Can you work these out from the model? Positions are in its coordinate system, mm. Face numbers are marked on the shaded views. A direction names the side the tool comes from. Give positions to 0.01 mm unless a question says otherwise; leave off trailing zeros. Loops run counter-clockwise (first coordinate to the right, second up) from the corner with the lowest first, then second, coordinate; pieces in that order, holes last. Notation, with made-up numbers: M 33,-6.5 L 58,-6.5 A24 ccw 58,7.5 Z; hole C 19.5,46 d8. An arc over 180 degrees is marked long. Put each result on its own line as item: value. Start each with the question number.
1) For P1, Ø8, axis at x = 21.5, y = 3.5, coming from the +Z side; P2, Ø3, axis at x = -3.5, y = 12, coming from the +Z side; P3, Ø5, axis at x = -26, z = -51, coming from the +Y side; P4, Ø2.5, axis at x = -28, z = -27.5, coming from the +Y side, each with a flat end and sliding along its axis, tell me the tip position at first contact or that it passes through.
2) If we mould it in two halves opening along X, with no side actions, what happens to the marked faces 4, 5 and 6? For each: +X half, -X half, draft (parallel to the pull), parting line (faces both ways), or undercut.
3) Please list where these lines run through material, in increasing order: line 1 along Z through (x, y) = (0, 2.75); line 2 along Z through (x, y) = (-27.5, 6.85); line 3 along Z through (x, y) = (4, 7.25). Write a range as from..to.
4) Imagine slicing it at A-A (y = 11.5). Write out the boundary of the cut face in (x, z).
5) For the marked faces 1, 2 and 3, which set-ups out of +Z, -Z, +X, -X, +Y, -Y let a thin tool reach every point of the face, with its end or its side?
6) Imagine slicing it at C-C (y = 5.25). State how many separate pieces and enclosed holes the cut face has, then the cut area to 3 significant figures.
7) Imagine slicing it at B-B (x = 18.5). Write out the boundary of the cut face in (y, z), then the cut area to 3 significant figures.
from build123d import *

# Parameters (mm, degrees)
BOSS_EXTRUDE1_DEPTH       = 7
FILLET1_R                 = 2
FILLET2_R                 = 10
SKETCH2_R                 = 10
BOSS_EXTRUDE2_DEPTH       = 8
FILLET3_R                 = 2
M10_CLEARANCE_HOLE1_D     = 10
M10_CLEARANCE_HOLE1_DEPTH = 10
M10_CLEARANCE_HOLE1_TIP   = 3.004303095
M5X0_8_TAPPED_HOLE1_D     = 4.2
M5X0_8_TAPPED_HOLE1_DEPTH = 12.4
M5X0_8_TAPPED_HOLE1_TIP   = 1.2618073
SKETCH6_R                 = 4.65
CUT_EXTRUDE1_DEPTH        = 0.55
SKETCH8_R                 = 4.65
CUT_EXTRUDE2_DEPTH        = 0.55
SKETCH9_R                 = 2.5
SKETCH10_R                = 4.65
CUT_EXTRUDE3_DEPTH        = 0.55
SKETCH11_R                = 2.5
SKETCH12_R                = 4.65
CUT_EXTRUDE4_DEPTH        = 0.55
SKETCH13_R                = 2.5


with BuildPart() as part:
    # Sketch1 → Boss-Extrude1 (new body)
    with BuildSketch(Plane(origin=(0, 0, 0), x_dir=(1, 0, 0), z_dir=(0, 1, 0))):
        with BuildLine():
            Line((-29, 35.312691864), (-29, 61.312691864))
            ThreePointArc((-29, 61.312691864), (-35.104593263, 71.654789625), (-24.072111437, 76.399195782))
            ThreePointArc((-24.072111437, 76.399195782), (0, 91.170808686), (24.072111437, 76.399195782))
            ThreePointArc((24.072111437, 76.399195782), (35.104593263, 71.654789625), (29, 61.312691864))
            Line((29, 61.312691864), (29, 35.312691864))
            ThreePointArc((29, 35.312691864), (35.126764687, 25.039526301), (24.203518415, 20.16532205))
            ThreePointArc((24.203518415, 20.16532205), (0, 5.30985101), (-24.203518415, 20.16532205))
            ThreePointArc((-24.203518415, 20.16532205), (-35.126764687, 25.039526301), (-29, 35.312691864))
        make_face()
    extrude(amount=BOSS_EXTRUDE1_DEPTH)

    # Fillet1
    fillet1_edges = [part.edges().sort_by_distance(p)[0] for p in [
        (29, 3.5, -61.312691864),
        (29, 3.5, -35.312691864),
        (-29, 3.5, -35.312691864),
        (-29, 3.5, -61.312691864),
    ]]
    fillet(fillet1_edges, radius=FILLET1_R)

    # Fillet2
    fillet2_edges = [part.edges().sort_by_distance(p)[0] for p in [
        (24.072111437, 3.5, -76.399195782),
        (24.203518415, 3.5, -20.16532205),
        (-24.203518415, 3.5, -20.16532205),
        (-24.072111437, 3.5, -76.399195782),
    ]]
    fillet(fillet2_edges, radius=FILLET2_R)

    # Sketch2 → Boss-Extrude2 (add)
    with BuildSketch(Plane(origin=(0, 7, 0), x_dir=(1, 0, 0), z_dir=(0, 1, 0))):
        with Locations(Location((0, 64.170808686, 0), (0, 0, 270))):
            Circle(SKETCH2_R)
        with Locations(Location((0, 32.454575041, 0), (0, 0, 270))):
            Circle(SKETCH2_R)
    extrude(amount=BOSS_EXTRUDE2_DEPTH)

    # Fillet3
    fillet3_edges = [part.edges().sort_by_distance(p)[0] for p in [
        (0, 7, -74.170808686),
        (0, 15, -74.170808686),
        (0, 7, -42.454575041),
        (0, 15, -42.454575041),
    ]]
    fillet(fillet3_edges, radius=FILLET3_R)

    # M10 Clearance Hole1
    with Locations(Plane(origin=(0, 0, -32.454575041), x_dir=(0, 0, -1), z_dir=(0, -1, 0))):
        with Locations((0, 0), (31.716233645, 0)):
            Hole(M10_CLEARANCE_HOLE1_D / 2, depth=M10_CLEARANCE_HOLE1_DEPTH)
            with Locations((0, 0, -(M10_CLEARANCE_HOLE1_DEPTH + M10_CLEARANCE_HOLE1_TIP / 2))):  # 118° drill point
                Cone(0, M10_CLEARANCE_HOLE1_D / 2, M10_CLEARANCE_HOLE1_TIP, mode=Mode.SUBTRACT)

    # M5x0.8 Tapped Hole1
    with Locations(Plane(origin=(-27.5, 7, -69.170808686), x_dir=(0, 0, 1), z_dir=(0, 1, 0))):
        with Locations((0, 0), (0, 55), (41.716233645, 55), (41.716233645, 0)):
            Hole(M5X0_8_TAPPED_HOLE1_D / 2, depth=M5X0_8_TAPPED_HOLE1_DEPTH)
            with Locations((0, 0, -(M5X0_8_TAPPED_HOLE1_DEPTH + M5X0_8_TAPPED_HOLE1_TIP / 2))):  # 118° drill point
                Cone(0, M5X0_8_TAPPED_HOLE1_D / 2, M5X0_8_TAPPED_HOLE1_TIP, mode=Mode.SUBTRACT)

    # Sketch6 → Cut-Extrude1 (cut)
    with BuildSketch(Plane(origin=(0, 7, 0), x_dir=(1, 0, 0), z_dir=(0, 1, 0))):
        with Locations(Location((27.5, 69.170808686, 0), (0, 0, 270))):
            Circle(SKETCH6_R)
    extrude(amount=-CUT_EXTRUDE1_DEPTH, mode=Mode.SUBTRACT)

    # Cut-Loft1: read off the stored shape, not the designer's step
    # Cut-Loft1: loft between two sections, ruled curve by curve
    cut_loft1_from = [
        Edge.make_bspline([(25.414803916, 4.3, -70.549923363), (22.656574563, 4.3, -66.379531195), (26.826966731, 4.3, -63.621301842), (29.585196084, 4.3, -67.79169401), (32.343425437, 4.3, -71.962086178), (28.173033269, 4.3, -74.720315531), (25.414803916, 4.3, -70.549923363)], [0, 0, 0, 0, 0.5, 0.5, 0.5, 1, 1, 1, 1], 3, [1, 0.333333333, 0.333333333, 1, 0.333333333, 0.333333333, 1]),
    ]
    cut_loft1_to = [
        Edge.make_bspline([(23.222066223, 6.45, -70.993384502), (19.576914593, 6.45, -62.437516949), (28.132782146, 6.45, -58.792365318), (31.777933777, 6.45, -67.348232871), (35.423085407, 6.45, -75.904100424), (26.867217854, 6.45, -79.549252055), (23.222066223, 6.45, -70.993384502)], [0, 0, 0, 0, 0.5, 0.5, 0.5, 1, 1, 1, 1], 3, [1, 0.333333333, 0.333333333, 1, 0.333333333, 0.333333333, 1]),
    ]
    cut_loft1 = Solid(Shell([*[Face.make_surface_from_curves(cut_loft1_from[k], cut_loft1_to[k]) for k in range(1)], Face(Wire(cut_loft1_from)), Face(Wire(cut_loft1_to))]))
    add(cut_loft1, mode=Mode.SUBTRACT)

    # Sketch8 → Cut-Extrude2 (cut)
    with BuildSketch(Plane(origin=(0, 7, 0), x_dir=(1, 0, 0), z_dir=(0, 1, 0))):
        with Locations(Location((-27.5, 69.170808686, 0), (0, 0, 270))):
            Circle(SKETCH8_R)
    extrude(amount=-CUT_EXTRUDE2_DEPTH, mode=Mode.SUBTRACT)

    # Sketch9 → section 0 of cut_loft2
    with BuildSketch(Plane(origin=(0, 4.3, 0), x_dir=(1, 0, 0), z_dir=(0, 1, 0)), mode=Mode.PRIVATE) as cut_loft2_s0:
        with Locations((-27.5, 69.170808686)):
            Circle(SKETCH9_R)
    # loft up to a face of the part (cut_loft2)
    loft([cut_loft2_s0.sketch, Face(Wire([part.edges().sort_by_distance((-24.110295882, 6.45, -72.353952729))[0]]))], mode=Mode.SUBTRACT)

    # Sketch10 → Cut-Extrude3 (cut)
    with BuildSketch(Plane(origin=(0, 7, 0), x_dir=(1, 0, 0), z_dir=(0, 1, 0))):
        with Locations(Location((-27.5, 27.454575041, 0), (0, 0, 270))):
            Circle(SKETCH10_R)
    extrude(amount=-CUT_EXTRUDE3_DEPTH, mode=Mode.SUBTRACT)

    # Sketch11 → section 0 of cut_loft3
    with BuildSketch(Plane(origin=(0, 4.3, 0), x_dir=(1, 0, 0), z_dir=(0, 1, 0)), mode=Mode.PRIVATE) as cut_loft3_s0:
        with Locations((-27.5, 27.454575041)):
            Circle(SKETCH11_R)
    # loft up to a face of the part (cut_loft3)
    loft([cut_loft3_s0.sketch, Face(Wire([part.edges().sort_by_distance((-24.110295882, 6.45, -30.637719083))[0]]))], mode=Mode.SUBTRACT)

    # Sketch12 → Cut-Extrude4 (cut)
    with BuildSketch(Plane(origin=(0, 7, 0), x_dir=(1, 0, 0), z_dir=(0, 1, 0))):
        with Locations(Location((27.5, 27.454575041, 0), (0, 0, 270))):
            Circle(SKETCH12_R)
    extrude(amount=-CUT_EXTRUDE4_DEPTH, mode=Mode.SUBTRACT)

    # Sketch13 → section 0 of cut_loft4
    with BuildSketch(Plane(origin=(0, 4.3, 0), x_dir=(1, 0, 0), z_dir=(0, 1, 0)), mode=Mode.PRIVATE) as cut_loft4_s0:
        with Locations((27.5, 27.454575041)):
            Circle(SKETCH13_R)
    # loft up to a face of the part (cut_loft4)
    loft([cut_loft4_s0.sketch, Face(Wire([part.edges().sort_by_distance((30.889704118, 6.45, -30.637719083))[0]]))], mode=Mode.SUBTRACT)


solid = part.part
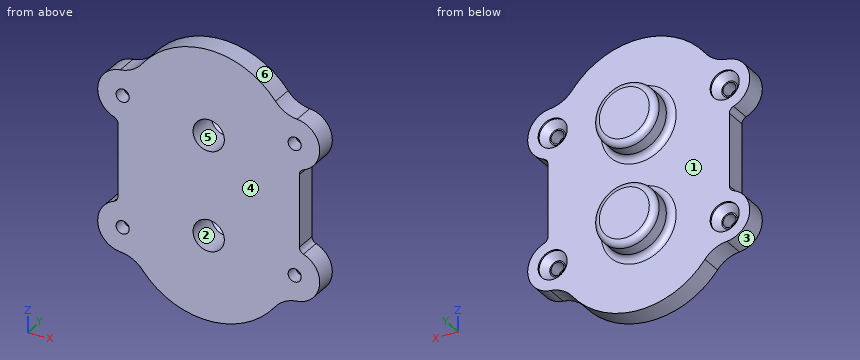
Recorded:
1. P1: z = -11.7
1. P2: z = -22.66
1. P3: y = 7
1. P4: through
2. face 4: draft
2. face 5: undercut
2. face 6: parting line
3. line 1: -91.17..-69.17, -59.17..-37.45, -27.45..-5.31
3. line 2: -77.22..-73.82, -64.52..-32.1, -22.8..-19.39
3. line 3: -74.45..-67.17, -61.17..-53.89, -42.74..-35.45, -29.45..-22.17
4. outline: C 0,-64.17 d20; C 0,-32.45 d20; hole C 0,-64.17 d5.01; hole C 0,-32.45 d5.01
5. face 1: +Y
5. face 2: -Y
5. face 3: -X, +Y, -Y
6. separate pieces: 1
6. enclosed holes: 6
6. area: 4,310 mm²
7. outline: M 0,-83.84 L 7,-83.84 L 7,-12.59 L 0,-12.59 Z
7. area: 499 mm²
